Geometry: see drawing. Coordinates: mm, zero at the bounding-box minimum. A direction names the side the tool comes from. Coordinates: 2 decimals unless noted, no trailing zeros. Order: outer loops, then holes, each group sorted by start corner. A loop starts at its lowest first (then second) coordinate and runs counter-clockwise, first axis right, second up.
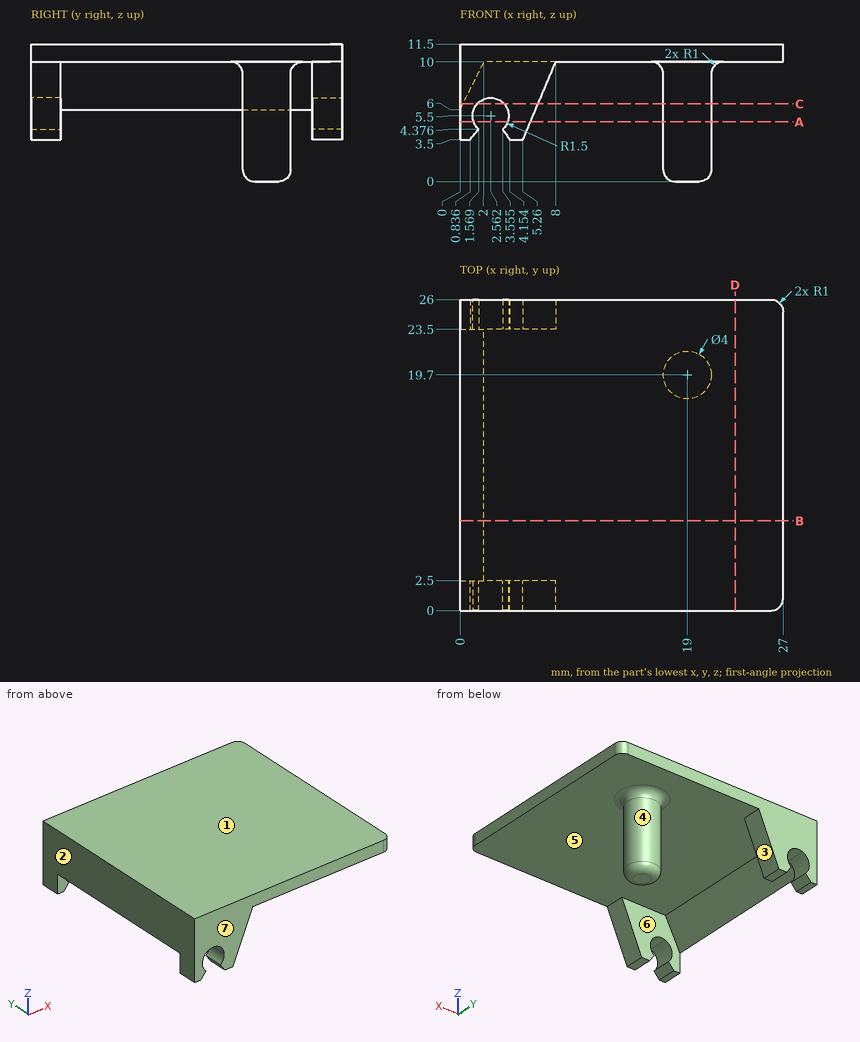
Q1. Pull-direction query (X, two-part tool) for the marked faces 1, 2, 3 and 4; classes: pulls with the +X half, pulls with the -X half, needs draft (parallel to the pull), parting line crosses it, or undercut.
Solutions:
face 1: needs draft
face 2: pulls with the -X half
face 3: pulls with the +X half
face 4: undercut
Q2. Section query C-C on z = 6.5. Give the number of separate pieces and of enclosed holes in the cut face.
Solutions:
separate pieces: 4
enclosed holes: 0
Q3. Material intervals for line 1 along Z through (x, y) = (23.25, 9); line 2 along Y through (x, z) = (2.75, 9); line 3 along X through (y, z) = (17, 8.5), sorted ascending.
Solutions:
line 1: z = 10 to 11.5
line 2: y = 0 to 2.5, 23.5 to 26
line 3: x = 0 to 1.25
Q4. Section query D-D on x = 23. Output: boundary loops of the cut face in (y, z).
Solutions:
outline: (0, 10) - (26, 10) - (26, 11.5) - (0, 11.5) - close
Q5. Pin query (flat end, axial travel): P1, Ø10, axis at x = 13.5, y = 16.5, coming from the -Z side; P2, Ø0.9, axis at x = 5, y = 1, coming from the -Z side; P3, Ø4, axis at x = 10.5, y = 15.5, coming from the -Z side. Return the tip coordinate at first contact, or that it passes through.
Solutions:
P1: stops at z = 0.07
P2: stops at z = 3.5
P3: stops at z = 10
Q6. Section query A-A on z = 5. Output: boundary loops of the cut face in (x, y).
Solutions:
outline: (0, 0) - (1.15, 0) - (1.15, 2.5) - (0, 2.5) - close; (0, 23.5) - (1.15, 23.5) - (1.15, 26) - (0, 26) - close; (3.98, 0) - (5.89, 0) - (5.89, 2.5) - (3.98, 2.5) - close; (3.98, 23.5) - (5.89, 23.5) - (5.89, 26) - (3.98, 26) - close; circle Ø4 at (19, 19.7)
Q7. Set-up query: the marked faces 5, 6 and 7. Return all of +Z, -Z, +X, -X, +Y, -Y with unobstructed straight access to the full face (end or side cutting, diameter ignored); none if empty.
Solutions:
face 5: -Z
face 6: -Z, +X
face 7: +Z, -Z, +X, -X, -Y
Q8. Section query B-B on y = 7.5. Output: boundary loops of the cut face in (x, z).
Solutions:
outline: (0, 6) - (2, 10) - (27, 10) - (27, 11.5) - (0, 11.5) - close
